Answer from the drawing. Dimensions are ordinates in mm from the lowest x, y and z of the part. A direction names the side the tool comes from. Give positions to 0.01 mm unless a question says otherwise; leave off trailing zeros. Loops run counter-clockwise (first coordinate to the right, second up) from the corner with the lowest first, then second, coordinate; pieces in that order, holes last.
Item 1: Section A-A, the plane x = 57.5 is taken. Give the vertices of the cut face in (y, z), and give its area (3 significant figures).
Item 2: A tool of negligible diameter and unlimited length cuts with its end or side. For the marked faces 1 and 2, from which of +Z, -Z, +X, -X, +Y, -Y can it reach the whole face along a straight path? Write none if from no direction.
Item 3: Section B-B, the plane z = 57.5 is taken. Give the vertices of the cut face in (x, y).
Item 4: Each of these flat-tipped pins is pushed along its axis until it touches: pin 1 Ø5 at (x, y) = (101, 13) entering from +Z; pin 2 Ø5 at (x, z) = (97, 102) entering from -Y; pin 3 Ø3 at (x, z) = (85.5, 60) entering from -Y; pin 4 Ø12 at (x, z) = (15.5, 42.5) entering from -Y. Where does it stop, or does it pass through?
Item 5: Consider line 1 along X through (y, z) = (21.25, 57.5); line 2 along Z through (x, y) = (57, 8); line 3 along X through (y, z) = (12, 57.5). Determine where each line is inside the solid, lowest interval first.
Item 6: Section C-C, the plane y = 2 is taken. Give the vertices of the cut face in (x, z), and give its area (3 significant figures).
Item 7: The mould has two halves that part along Z. Classify the marked faces 3, 4 and 5: pulls with the +Z half, pulls with the -Z half, needs draft (parallel to the pull), parting line crosses it, or undercut.
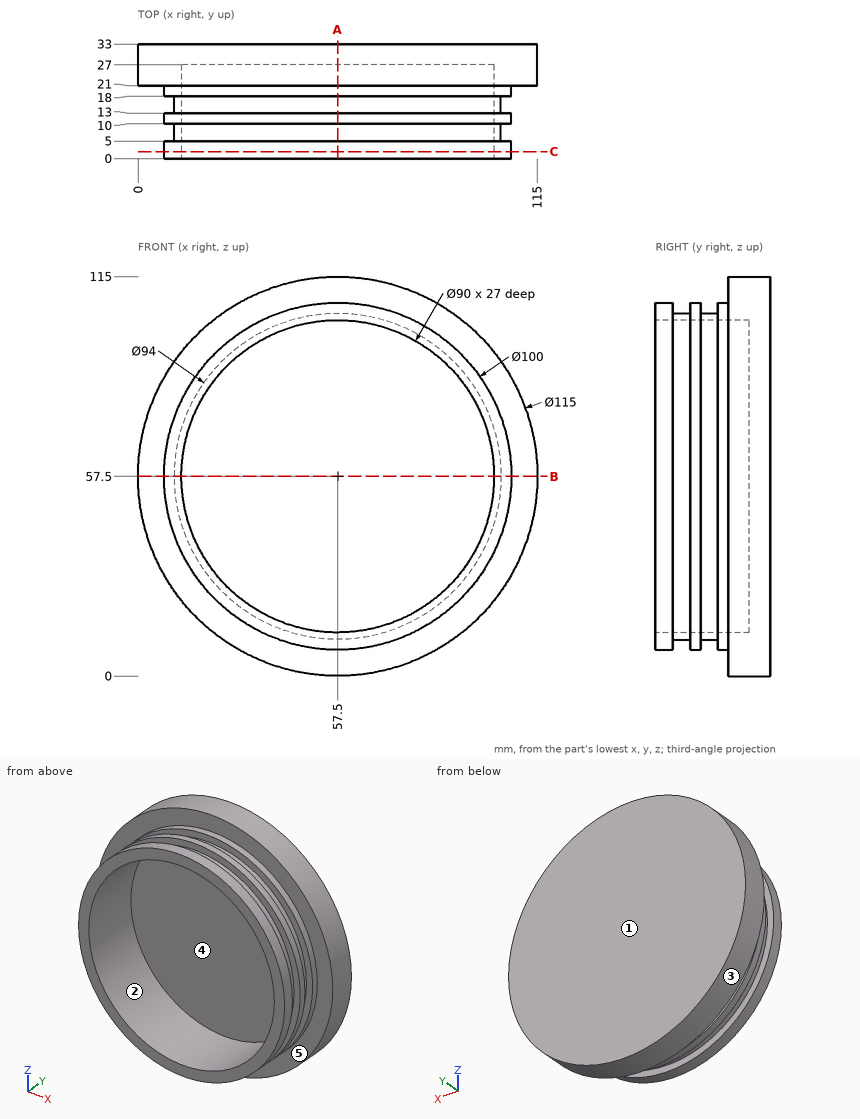
Worked answers:
1. outline: (0, 7.5) - (5, 7.5) - (5, 10.5) - (10, 10.5) - (10, 7.5) - (13, 7.5) - (13, 10.5) - (18, 10.5) - (18, 7.5) - (21, 7.5) - (21, 0) - (33, 0) - (33, 115) - (21, 115) - (21, 107.5) - (18, 107.5) - (18, 104.5) - (13, 104.5) - (13, 107.5) - (10, 107.5) - (10, 104.5) - (5, 104.5) - (5, 107.5) - (0, 107.5) - (0, 102.5) - (27, 102.5) - (27, 12.5) - (0, 12.5) - close
1. area: 990 mm2
2. face 1: +Z, -Z, +X, -X, +Y
2. face 2: -Y
3. outline: (0, 21) - (7.5, 21) - (7.5, 18) - (10.5, 18) - (10.5, 13) - (7.5, 13) - (7.5, 10) - (10.5, 10) - (10.5, 5) - (7.5, 5) - (7.5, 0) - (12.5, 0) - (12.5, 27) - (102.5, 27) - (102.5, 0) - (107.5, 0) - (107.5, 5) - (104.5, 5) - (104.5, 10) - (107.5, 10) - (107.5, 13) - (104.5, 13) - (104.5, 18) - (107.5, 18) - (107.5, 21) - (115, 21) - (115, 33) - (0, 33) - close
4. pin 1: stops at z = 86.12
4. pin 2: stops at y = 21
4. pin 3: stops at y = 27
4. pin 4: stops at y = 0
5. line 1: x = 0 to 12.5, 102.5 to 115
5. line 2: z = 10.5 to 12.5, 102.5 to 104.5
5. line 3: x = 7.5 to 12.5, 102.5 to 107.5
6. outline: circle Ø100 at (57.5, 57.5); hole circle Ø90 at (57.5, 57.5)
6. area: 1,490 mm2
7. face 3: parting line crosses it
7. face 4: undercut
7. face 5: needs draft
